```python
from build123d import *

# Parameters (mm, degrees)
SKETCH1_W           = 64
SKETCH1_H           = 153
SKETCH1_R           = 2.1
BOSS_EXTRUDE1_DEPTH = 3
FILLET2_R           = 0.5
FILLET3_R           = 1


with BuildPart() as part:
    # Sketch1 → Boss-Extrude1 (new body)
    with BuildSketch(Plane.XY):
        with Locations((28.5, -56.5)):
            Rectangle(SKETCH1_W, SKETCH1_H)
        with Locations((8.5, 11)):
            Circle(SKETCH1_R, mode=Mode.SUBTRACT)
        with Locations(Location((48.5, 11, 0), (0, 0, 180))):
            Circle(SKETCH1_R, mode=Mode.SUBTRACT)
        with Locations((48.5, -127)):
            Circle(SKETCH1_R, mode=Mode.SUBTRACT)
        with Locations(Location((8.5, -127, 0), (0, 0, 180))):
            Circle(SKETCH1_R, mode=Mode.SUBTRACT)
        with BuildLine():
            Line((0, 0), (23.455727081, 0))
            ThreePointArc((23.455727081, 0), (24.673249939, -0.413293319), (25.387578733, -1.48236191))
            Line((25.387578733, -1.48236191), (26.702101743, -6.388228568))
            ThreePointArc((26.702101743, -6.388228568), (27.237848338, -7.19003001), (28.150990482, -7.5))
            Line((28.150990482, -7.5), (28.849009518, -7.5))
            ThreePointArc((28.849009518, -7.5), (29.762151662, -7.19003001), (30.297898257, -6.388228568))
            Line((30.297898257, -6.388228568), (31.612421267, -1.48236191))
            ThreePointArc((31.612421267, -1.48236191), (32.326750061, -0.413293319), (33.544272919, 0))
            Line((33.544272919, 0), (57, 0))
            Line((57, 0), (57, -108))
            Line((57, -108), (0, -108))
            Line((0, -108), (0, 0))
        make_face(mode=Mode.SUBTRACT)
    extrude(amount=BOSS_EXTRUDE1_DEPTH)

    # Fillet2
    fillet2_edges = [part.edges().sort_by_distance(p)[0] for p in [
        (-3.5, 20, 1.5),
        (60.5, 20, 1.5),
        (60.5, -133, 1.5),
        (-3.5, -133, 1.5),
    ]]
    fillet(fillet2_edges, radius=FILLET2_R)

    # Fillet3
    fillet3_edges = [part.edges().sort_by_distance(p)[0] for p in [
        (0, 0, 1.5),
        (0, -108, 1.5),
        (57, -108, 1.5),
        (57, 0, 1.5),
    ]]
    fillet(fillet3_edges, radius=FILLET3_R)


solid = part.part
```
Part model, mm, in its own coordinate system. A direction names the side the tool comes from. Round coordinates to 2 decimals unless told otherwise and drop trailing zeros. Loops run counter-clockwise (first coordinate to the right, second up) from the corner with the lowest first, then second, coordinate; pieces in that order, holes last. Notation, with made-up numbers: (39.5, 36) -> (50.5, 36) arc R33 ccw to (50.5, 70) -> close; hole circle Ø11 at (-38, 78). An arc over 180 degrees is marked (long way). Use a Markdown table: item, result.
1) Cut at A-A, the plane x = 8.5. List the corners of the cut face in (y, z), and give its area (3 significant figures).
The answers:
| item | result |
|---|---|
| outline | (-133, 0) -> (-129.1, 0) -> (-129.1, 3) -> (-133, 3) -> close; (-124.9, 0) -> (-108, 0) -> (-108, 3) -> (-124.9, 3) -> close; (0, 0) -> (8.9, 0) -> (8.9, 3) -> (0, 3) -> close; (13.1, 0) -> (20, 0) -> (20, 3) -> (13.1, 3) -> close |
| area | 110 mm2 |
2) Pull direction Y, two halves, no side cores. Call faces 1 (the cylindrical face through (49.469, -128.863, 1.479)), 2 (the flat face through (60.5, -58, 1)), 3 (the flat face through (30.946, -3.97, 1.479)), 4 (the flat face through (28, 20, 1)): pulls with the +Y half, pulls with the -Y half, needs draft (parallel to the pull), parting line crosses it, or undercut.
The answers:
| item | result |
|---|---|
| face 1 | undercut |
| face 2 | needs draft |
| face 3 | undercut |
| face 4 | pulls with the +Y half |
3) Probe line 1 (Y direction, x = 8.5, z = 1.6); line 2 (X direction, y = -55, z = 1.2); line 3 (Y direction, x = 16.5, z = 2.05). List the from-to ranges inside material, lowest first. Write a range as [from, to].
The answers:
| item | result |
|---|---|
| line 1 | y = [-133, -129.1], [-124.9, -108], [0, 8.9], [13.1, 20] |
| line 2 | x = [-3.5, 0], [57, 60.5] |
| line 3 | y = [-133, -108], [0, 20] |
4) Cut at D-D, the plane y = -16.5. List the corners of the cut face in (x, z), and give its area (3 significant figures).
The answers:
| item | result |
|---|---|
| outline | (-3.5, 0) -> (0, 0) -> (0, 3) -> (-3.5, 3) -> close; (57, 0) -> (60.5, 0) -> (60.5, 3) -> (57, 3) -> close |
| area | 21.0 mm2 |
5) Tool access for faces 5 (the flat face through (45, 0, 1)), 6 (the flat face through (-2, -62, 3)): list every direction of +Z, -Z, +X, -X, +Y, -Y with a clear straight run to the whole face (end or side of a thin tool).
The answers:
| item | result |
|---|---|
| face 5 | +Z, -Z |
| face 6 | +Z, +X, -X, +Y, -Y |
6) Cut at C-C, the plane z = 1.35. List the corners of the cut face in (x, y), and give its area (3 significant figures).
The answers:
| item | result |
|---|---|
| outline | (-3.5, -132.5) arc R0.5 ccw to (-3, -133) -> (60, -133) arc R0.5 ccw to (60.5, -132.5) -> (60.5, 19.5) arc R0.5 ccw to (60, 20) -> (-3, 20) arc R0.5 ccw to (-3.5, 19.5) -> close; hole (0, -107) arc R1 ccw to (1, -108) -> (56, -108) arc R1 ccw to (57, -107) -> (57, -1) arc R1 ccw to (56, 0) -> (33.54, 0) arc R2 ccw to (31.61, -1.48) -> (30.3, -6.39) arc R1.5 cw to (28.85, -7.5) -> (28.15, -7.5) arc R1.5 cw to (26.7, -6.39) -> (25.39, -1.48) arc R2 ccw to (23.46, 0) -> (1, 0) arc R1 ccw to (0, -1) -> close; hole circle Ø4.2 at (8.5, -127); hole circle Ø4.2 at (8.5, 11); hole circle Ø4.2 at (48.5, -127); hole circle Ø4.2 at (48.5, 11) |
| area | 3,620 mm2 |
7) Cut at B-B, the plane y = -127. List the corners of the cut face in (x, z), and give its area (3 significant figures).
The answers:
| item | result |
|---|---|
| outline | (-3.5, 0) -> (6.4, 0) -> (6.4, 3) -> (-3.5, 3) -> close; (10.6, 0) -> (46.4, 0) -> (46.4, 3) -> (10.6, 3) -> close; (50.6, 0) -> (60.5, 0) -> (60.5, 3) -> (50.6, 3) -> close |
| area | 167 mm2 |
